For this review, take the finished solid that the model builds, in its own axes (mm). Face numbers are marked on the shaded views. Round coordinates to 2 decimals unless told otherwise and drop trailing zeros. Answer as CSV lines item,"result". Start each with the question number.
Item 1: Mouldability with a two-part tool opening along Y and no side actions: class the marked faces 1 and 2 as +Y half, -Y half, draft (parallel to the pull), parting line (faces both ways), or undercut.
Item 2: For pin 1 Ø4 at (x, z) = (-184.15, 50.8) entering from -Y; pin 2 Ø5.5 at (x, y) = (-446, 6.5) entering from +Z; pin 3 Ø9.5 at (y, z) = (14, 53.5) entering from -X, all flat-tipped, find the tip position at first contact; note any pin that passes through.
Item 3: Wall thickness on probe 1 along Z at (x, y) = (-361.95, 8.5); probe 2 along X at (y, z) = (18, 52); probe 3 along X at (y, z) = (11.25, 39.5): over which ranges is each line inside the solid? List them lowest first. Write a range as from..to.
```python
from build123d import *

# Parameters (mm, degrees)
F0_W     = 914.4
F0_H     = 127
F1_DEPTH = 19.05
F2_W     = 19.05
F2_H     = 25.4
F3_DEPTH = 19.051
F5_D     = 4.7625


with BuildPart() as f1:
    # F0 (on Front) → F1 (new body)
    with BuildSketch(Plane.XZ):
        Rectangle(F0_W, F0_H)
    extrude(amount=-F1_DEPTH)

    # F2 (on face) → F3 (cut, through all)
    with BuildSketch(Plane.XZ):
        with Locations((-447.675, 50.8)):
            Rectangle(F2_W, F2_H)
        with Locations((447.675, 50.8)):
            Rectangle(F2_W, F2_H)
    extrude(amount=-F3_DEPTH, mode=Mode.SUBTRACT)

    # F5 (through all)
    with Locations(Plane.XZ):
        with Locations((-361.95, 50.8), (-184.15, 50.8), (-6.35, 50.8), (171.45, 50.8), (349.25, 50.8)):
            Hole(F5_D / 2)


solid = f1.part
```
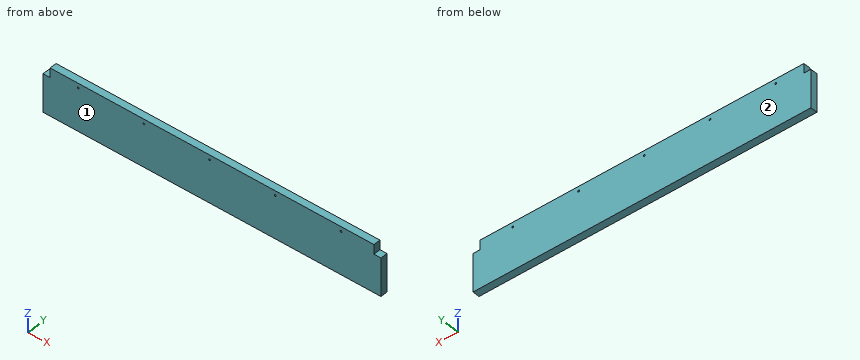
Output values:
1,face 1,"-Y half"
1,face 2,"+Y half"
2,pin 1,"passes through"
2,pin 2,"stops at z = 38.1"
2,pin 3,"stops at x = -438.15"
3,probe 1,"z = -63.5..48.42, 53.18..63.5"
3,probe 2,"x = -438.15..-364.01, -359.89..-186.21, -182.09..-8.41, -4.29..169.39, 173.51..347.19, 351.31..438.15"
3,probe 3,"x = -438.15..438.15"
